For this review, take the finished solid that the model builds, in its own axes (mm). A direction names the side the tool comes from. Give positions to 0.01 mm unless a question says otherwise; leave off trailing zeros. Loops run counter-clockwise (first coordinate to the right, second up) from the corner with the lowest first, then second, coordinate; pieces in that order, holes last. Notation, with made-up numbers: (-3, 27) -> (22, 27) arc R24 ccw to (22, 64) -> close; hole circle Ø10 at (48.5, -29.5). An arc over 180 degrees is marked (long way). Write each question's results on one line, items separated by ' | '. Start each with the question number.
```python
from build123d import *

# Parameters (mm, degrees)
SKETCH_1_R          = 5.5
EXTRUDE_1_DEPTH     = 26
SKETCH_2_W          = 8
SKETCH_2_H          = 18
CUT_EXTRUDE_1_DEPTH = 25
SKETCH_3_R          = 1.5
CUT_EXTRUDE_2_DEPTH = 25
CUT_EXTRUDE_3_DEPTH = 11


with BuildPart() as part:
    # 草图1 → 凸台-拉伸1 (new body)
    with BuildSketch(Plane(origin=(0, 0, 0), x_dir=(1, 0, 0), z_dir=(0, 1, 0))):
        Circle(SKETCH_1_R)
    extrude(amount=EXTRUDE_1_DEPTH)

    # 草图2 → 切除-拉伸1 (cut, symmetric)
    with BuildSketch(Plane.XY):
        with Locations((0, 26)):
            Rectangle(SKETCH_2_W, SKETCH_2_H)
    extrude(amount=CUT_EXTRUDE_1_DEPTH, both=True, mode=Mode.SUBTRACT)

    # 草图3 → 切除-拉伸2 (cut, symmetric)
    with BuildSketch(Plane(origin=(-4, 0, 0), x_dir=(0, 0, -1), z_dir=(1, 0, 0))):
        with Locations((0, 23)):
            Circle(SKETCH_3_R)
    extrude(amount=CUT_EXTRUDE_2_DEPTH, both=True, mode=Mode.SUBTRACT)

    # 草图5 → 切除-拉伸3 (cut, symmetric)
    with BuildSketch(Plane(origin=(0, 0, 0), x_dir=(0, 0, -1), z_dir=(1, 0, 0))):
        with BuildLine():
            Line((-4.153311931, 21.5), (-12.215121886, 24.91830584))
            Line((-12.215121886, 24.91830584), (0.629850505, 32.78071868))
            Line((0.629850505, 32.78071868), (12.991410006, 24.598657791))
            Line((12.991410006, 24.598657791), (4.153311931, 21.5))
            ThreePointArc((4.153311931, 21.5), (0, 25.653311931), (-4.153311931, 21.5))
        make_face()
    extrude(amount=CUT_EXTRUDE_3_DEPTH, both=True, mode=Mode.SUBTRACT)


solid = part.part
```
1. For pin 1 Ø5 at (x, z) = (-3.5, -4) entering from +Y; pin 2 Ø6 at (x, z) = (-0.5, 0.5) entering from +Y; pin 3 Ø2.5 at (y, z) = (23, 0) entering from -X, all flat-tipped, find the tip position at first contact; note any pin that passes through.
2. Machinability: for faces 1 (the flat face through (4, 20, 0)), 2 (the cylindrical face through (-4.74, 23.45, -1.43)), which of the approach directions +Z, -Z, +X, -X, +Y, -Y give a long, thin tool a straight path to every point of the face, cutting with its end or side? Answer none if there is none.
3. We need section B-B (y = 21.25). Write out the cut boundary in (x, z), plus the area to 3 significant figures.
4. Wall thickness on L1, parallel to Y at x = -4.45, z = 0; L2, parallel to Y at x = -2, z = 4.75; L3, parallel to Z at x = 4.4, y = 23: over which ranges is each line inside the solid? List them lowest first.
5. We need section C-C (x = -4.5). Write out the cut boundary in (y, z), plus the area to 3 significant figures.
6. Draft analysis for pull direction X (two halves, no side actions). For faces 3 (the flat face through (0, 17, 0)), 4 (the flat face through (0, 0, 0)), 5 (the cylindrical face through (5.246, 9.806, -1.652)), state which applies: released by +X, released by -X, zero draft, split by the parting line, or undercut.
7. We need section D-D (y = 10). Write out the cut boundary in (x, z).
8. We need section A-A (z = -1). Write out the cut boundary in (x, y).
Response:
1) pin 1: stops at y = 25.35 | pin 2: stops at y = 17 | pin 3: passes through
2) face 1: +Z, -Z, +Y | face 2: +X, -X
3) outline: (-4, -3.77) -> (-4, 3.77) arc R5.5 ccw to start; (4, -3.77) arc R5.5 ccw to (4, 3.77) -> close | area: 15.6 mm2
4) L1: y = 0 to 21.5, 24.5 to 25.65 | L2: y = 0 to 17 | L3: z = -3.3 to -1.5, 1.5 to 3.3
5) outline: (0, -3.16) -> (24.19, -3.16) arc R4.15 ccw to (24.19, 3.16) -> (0, 3.16) -> close; hole circle Ø3 at (23, 0) | area: 152 mm2
6) face 3: undercut | face 4: zero draft | face 5: split by the parting line
7) outline: circle Ø11 at (0, 0)
8) outline: (-5.41, 0) -> (5.41, 0) -> (5.41, 21.88) -> (4, 21.88) -> (4, 17) -> (-4, 17) -> (-4, 21.88) -> (-5.41, 21.88) -> close; (-5.41, 24.12) -> (-4, 24.12) -> (-4, 25.53) -> (-5.41, 25.53) -> close; (4, 24.12) -> (5.41, 24.12) -> (5.41, 25.53) -> (4, 25.53) -> close
